Here's the drawing with two shaded views (mm, measured from the low corner). I have some questions. Round coordinates to 2 decimals unless told otherwise and drop trailing zeros. Loops run counter-clockwise (first coordinate to the right, second up) from the corner with the lowest first, then second, coordinate; pieces in that order, holes last. Notation, with made-up numbers: (2.25, -34.5) -> (60.25, -34.5) arc R12 ccw to (60.25, -11.5) -> close; hole circle Ø4 at (81.25, 39.25). An arc over 180 degrees is marked (long way). Write item = value, one per line.
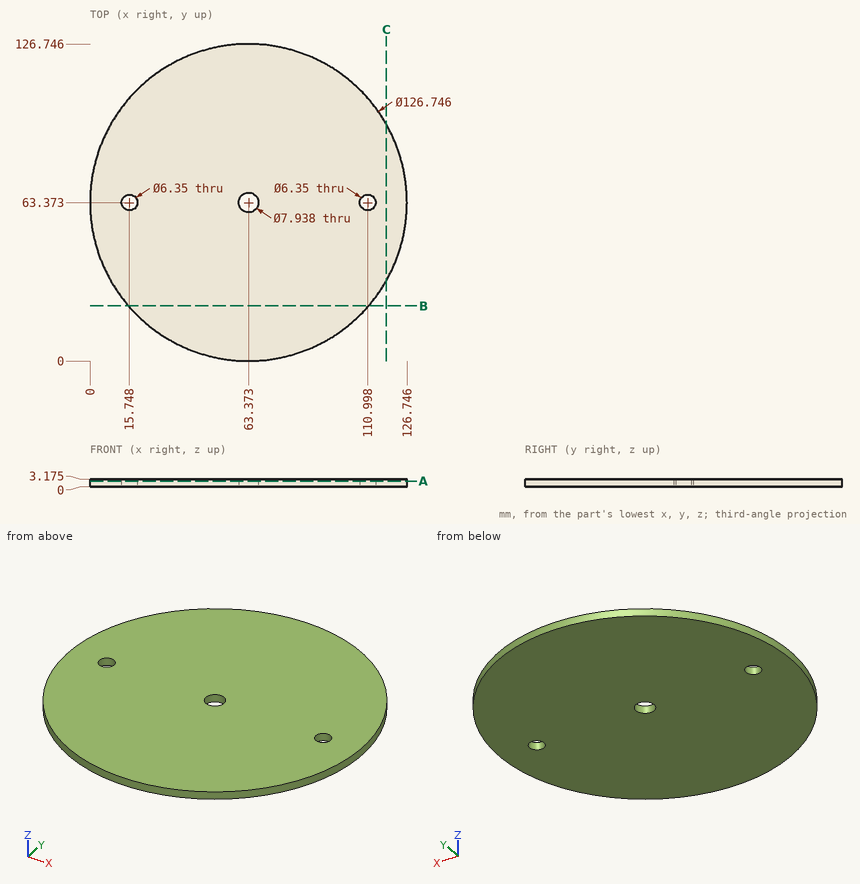
1. I need wall thicknesses on line 1 (Y direction, x = 25.5, z = 0.2) (1 decimal); line 2 (X direction, y = 60, z = 1.8) (1 decimal); line 3 (Y direction, x = 65, z = 2.45) (1 decimal). Which ranges of each line are inside material? Lowest first, please. Write a range as [from, to].
Entries:
line_1 = [12.6, 114.2]
line_2 = [0.1, 61.3], [65.5, 126.7]
line_3 = [0, 59.8], [67, 126.7]
2. Suppose I cut it at A-A, the plane z = 2.3. Count the separate pieces of the cut face and the enclosed holes in it, and give its area (3 significant figures).
Entries:
separate_pieces = 1
enclosed_holes = 3
area = 12,500 mm²
3. Suppose I cut it at B-B, the plane y = 22. List the corners of the cut face in (x, z) for me (1 decimal), and give its area (3 significant figures).
Entries:
outline = (15.4, 0) -> (111.4, 0) -> (111.4, 3.2) -> (15.4, 3.2) -> close
area = 305 mm²
4. I'm going to push flat-ended pins straight in: pin 1 (5 mm diameter, centred on x = 110.998, y = 63.373, fed in from -Z); pin 2 (1.5 mm diameter, centred on y = 86.5, z = 1.5, fed in from +X). Where does each tip first touch, or does it pass through?
Entries:
pin_1 = through
pin_2 = 122.66
5. Suppose I cut it at C-C, the plane x = 118.5. List the corners of the cut face in (y, z) for me (1 decimal).
Entries:
outline = (32.1, 0) -> (94.6, 0) -> (94.6, 3.2) -> (32.1, 3.2) -> close
